from build123d import *

# Parameters (mm, degrees)
BOSS_EXTRUDE1_DEPTH                                  = 3
FILLET1_R                                            = 5
CUT_EXTRUDE1_REACH                                   = 56.362
SKETCH5_W                                            = 36
SKETCH5_H                                            = 28
FILLET2_R                                            = 5
CSK_FOR_M2_5_COUNTERSUNK_FLAT_HEAD_SCREW_D           = 2.7
CSK_FOR_M2_5_COUNTERSUNK_FLAT_HEAD_SCREW_CSINK_D     = 5.5
CSK_FOR_M2_5_COUNTERSUNK_FLAT_HEAD_SCREW_CSINK_ANGLE = 90
CUT_EXTRUDE2_REACH                                   = 56.362
SKETCH3_R                                            = 2.5
MIRROR1_AT_THE_SECOND_PLANE_COPY_1_D                 = 2.7
MIRROR1_AT_THE_SECOND_PLANE_COPY_1_CSINK_D           = 5.5
MIRROR1_AT_THE_SECOND_PLANE_COPY_1_CSINK_ANGLE       = 90
MIRROR1_AT_THE_SECOND_PLANE_COPY_2_REACH             = 56.362
MIRROR1_AT_THE_SECOND_PLANE_COPY_2_SKETC_R           = 2.5
CUT_EXTRUDE3_REACH                                   = 56.362
SKETCH7_R                                            = 1
MIRROR2_AT_THE_SECOND_PLANE_COPY_1_REACH             = 56.362
MIRROR2_AT_THE_SECOND_PLANE_COPY_1_SKETC_R           = 1


with BuildPart() as part:
    # Sketch1 → Boss-Extrude1 (new body)
    with BuildSketch(Plane(origin=(0, 0, 0), x_dir=(1, 0, 0), z_dir=(0, 1, 0))):
        Polygon((8, 26), (-8, 26), (-8, 46.5), (-28, 46.5), (-28, -46.5), (-8, -46.5), (-8, -26), (8, -26), (8, -46.5), (28, -46.5), (28, 46.5), (8, 46.5), align=None)
    extrude(amount=BOSS_EXTRUDE1_DEPTH)

    # Fillet1
    fillet1_edges = [part.edges().sort_by_distance(p)[0] for p in [
        (-8, 1.5, -26),
        (8, 1.5, -26),
        (8, 1.5, -46.5),
        (28, 1.5, -46.5),
        (28, 1.5, 46.5),
        (8, 1.5, 46.5),
        (8, 1.5, 26),
        (-8, 1.5, 26),
        (-8, 1.5, 46.5),
        (-28, 1.5, 46.5),
        (-28, 1.5, -46.5),
        (-8, 1.5, -46.5),
    ]]
    fillet(fillet1_edges, radius=FILLET1_R)

    # Sketch5 → Cut-Extrude1 (cut, up to next)
    with BuildSketch(Plane(origin=(0, 3, 0), x_dir=(1, 0, 0), z_dir=(0, 1, 0)), mode=Mode.PRIVATE) as cut_extrude1_sk1:
        Rectangle(SKETCH5_W, SKETCH5_H)
    cut_extrude1_tool1 = extrude(cut_extrude1_sk1.sketch, amount=-CUT_EXTRUDE1_REACH, mode=Mode.PRIVATE) & part.part
    add(cut_extrude1_tool1.solids().sort_by_distance((0, 3, 0))[0], mode=Mode.SUBTRACT)

    # Fillet2
    fillet2_edges = [part.edges().sort_by_distance(p)[0] for p in [
        (-18, 1.5, 14),
        (-18, 1.5, -14),
        (18, 1.5, -14),
        (18, 1.5, 14),
    ]]
    fillet(fillet2_edges, radius=FILLET2_R)

    # CSK for M2.5 Countersunk Flat Head Screw1 (through all)
    with Locations(Plane(origin=(-18, 3, -37), x_dir=(0, 0, 1), z_dir=(0, 1, 0))):
        with Locations((0, 0), (14, 0)):
            csk_for_m2_5_countersunk_flat_head_screw = CounterSinkHole(CSK_FOR_M2_5_COUNTERSUNK_FLAT_HEAD_SCREW_D / 2, CSK_FOR_M2_5_COUNTERSUNK_FLAT_HEAD_SCREW_CSINK_D / 2, counter_sink_angle=CSK_FOR_M2_5_COUNTERSUNK_FLAT_HEAD_SCREW_CSINK_ANGLE)

    # Sketch3 → Cut-Extrude2 (cut, up to next)
    with BuildSketch(Plane(origin=(0, 3, 0), x_dir=(1, 0, 0), z_dir=(0, 1, 0)), mode=Mode.PRIVATE) as cut_extrude2_sk1:
        with Locations(Location((-18, 30, 0), (0, 0, 270))):
            Circle(SKETCH3_R)
    cut_extrude2_tool1 = extrude(cut_extrude2_sk1.sketch, amount=-CUT_EXTRUDE2_REACH, mode=Mode.PRIVATE) & part.part
    cut_extrude2 = cut_extrude2_tool1.solids().sort_by_distance((-18, 3, -30))[0]
    add(cut_extrude2, mode=Mode.SUBTRACT)

    # Mirror1: CSK for M2.5 Countersunk Flat Head Screw1, Cut-Extrude2 across plane
    add(csk_for_m2_5_countersunk_flat_head_screw.mirror(Plane(origin=(0, 0, 0), x_dir=(0, 0, 1), z_dir=(1, 0, 0))), mode=Mode.SUBTRACT)
    add(cut_extrude2.mirror(Plane(origin=(0, 0, 0), x_dir=(0, 0, 1), z_dir=(1, 0, 0))), mode=Mode.SUBTRACT)

    # Mirror1 at the second plane: CSK for M2.5 Countersunk Flat Head Screw1, Cut-Extrude2 across plane
    add(csk_for_m2_5_countersunk_flat_head_screw.mirror(Plane.XY), mode=Mode.SUBTRACT)
    add(cut_extrude2.mirror(Plane.XY), mode=Mode.SUBTRACT)

    # Mirror1 at the second plane copy 1 (through all)
    with Locations(Plane(origin=(18, 3, 37), x_dir=(0, 0, -1), z_dir=(0, 1, 0))):
        with Locations((0, 0), (14, 0)):
            CounterSinkHole(MIRROR1_AT_THE_SECOND_PLANE_COPY_1_D / 2, MIRROR1_AT_THE_SECOND_PLANE_COPY_1_CSINK_D / 2, counter_sink_angle=MIRROR1_AT_THE_SECOND_PLANE_COPY_1_CSINK_ANGLE)

    # Mirror1 at the second plane copy 2 sketc → Mirror1 at the second plane copy 2 (cut, up to next)
    with BuildSketch(Plane(origin=(0, 3, 0), x_dir=(-1, 0, 0), z_dir=(0, 1, 0)), mode=Mode.PRIVATE) as mirror1_at_the_second_plane_copy_2_sk1:
        with Locations(Location((-18, 30, 0), (0, 0, 270))):
            Circle(MIRROR1_AT_THE_SECOND_PLANE_COPY_2_SKETC_R)
    mirror1_at_the_second_plane_copy_2_tool1 = extrude(mirror1_at_the_second_plane_copy_2_sk1.sketch, amount=-MIRROR1_AT_THE_SECOND_PLANE_COPY_2_REACH, mode=Mode.PRIVATE) & part.part
    add(mirror1_at_the_second_plane_copy_2_tool1.solids().sort_by_distance((18, 3, 30))[0], mode=Mode.SUBTRACT)

    # Sketch7 → Cut-Extrude3 (cut, up to next)
    with BuildSketch(Plane(origin=(0, 3, 0), x_dir=(1, 0, 0), z_dir=(0, 1, 0)), mode=Mode.PRIVATE) as cut_extrude3_sk1:
        with Locations(Location((-23.3, 10, 0), (0, 0, 270))):
            Circle(SKETCH7_R)
    cut_extrude3_tool1 = extrude(cut_extrude3_sk1.sketch, amount=-CUT_EXTRUDE3_REACH, mode=Mode.PRIVATE) & part.part
    cut_extrude3 = cut_extrude3_tool1.solids().sort_by_distance((-23.3, 3, -10))[0]
    add(cut_extrude3, mode=Mode.SUBTRACT)

    # Mirror2: Cut-Extrude3 across plane
    add(cut_extrude3.mirror(Plane(origin=(0, 0, 0), x_dir=(0, 0, 1), z_dir=(1, 0, 0))), mode=Mode.SUBTRACT)

    # Mirror2 at the second plane: Cut-Extrude3 across plane
    add(cut_extrude3.mirror(Plane.XY), mode=Mode.SUBTRACT)

    # Mirror2 at the second plane copy 1 sketc → Mirror2 at the second plane copy 1 (cut, up to next)
    with BuildSketch(Plane(origin=(0, 3, 0), x_dir=(-1, 0, 0), z_dir=(0, 1, 0)), mode=Mode.PRIVATE) as mirror2_at_the_second_plane_copy_1_sk1:
        with Locations(Location((-23.3, 10, 0), (0, 0, 270))):
            Circle(MIRROR2_AT_THE_SECOND_PLANE_COPY_1_SKETC_R)
    mirror2_at_the_second_plane_copy_1_tool1 = extrude(mirror2_at_the_second_plane_copy_1_sk1.sketch, amount=-MIRROR2_AT_THE_SECOND_PLANE_COPY_1_REACH, mode=Mode.PRIVATE) & part.part
    add(mirror2_at_the_second_plane_copy_1_tool1.solids().sort_by_distance((23.3, 3, 10))[0], mode=Mode.SUBTRACT)


solid = part.part
Verification items for the finished model (mm, model axes). A direction names the side the tool comes from. Round coordinates to 2 decimals unless told otherwise and drop trailing zeros. Write each loop counter-clockwise with the first axis right and the second up, starting at its lowest first coordinate (ties: lowest second). Pieces come first, ordered by that corner, then holes.
(1) Section check D-D (y = 1.05). Give the number of separate pieces and of enclosed holes in the cut face, plus the area to 3 significant figures.
Returned:
separate pieces: 1
enclosed holes: 17
area: 3,410 mm2
(2) Access from +Z, -Z, +X, -X, +Y, -Y to the whole of each face (thin tool, end or side, straight path). Record for faces 4 (the cylindrical face through (-26.57, 1.52, 45)), 5 (the flat face through (18, 2, 0)), 6 (the flat face through (0, 1, 26)).
Returned:
face 4: +Z, -X, +Y, -Y
face 5: +Y, -Y
face 6: +Z, +Y, -Y
(3) Material ranges on line 1 (X direction, y = 0.35, z = 37); line 2 (X direction, y = 1.1, z = 23); line 3 (Z direction, x = 7, y = 0.75), recorded low to high.
Returned:
line 1: x = -28 to -19.35, -16.65 to -8, 8 to 16.65, 19.35 to 28
line 2: x = -28 to -19.35, -16.65 to 16.65, 19.35 to 28
line 3: z = -28 to -14, 14 to 28
(4) Section check B-B (x = 0). Enter the section's corners in (y, z).
Returned:
outline: (0, -26) - (3, -26) - (3, -14) - (0, -14) - close; (0, 14) - (3, 14) - (3, 26) - (0, 26) - close
(5) Mould release check, pull along Z, two halves, no side actions. Record for faces 1 (the cylindrical face through (-17.9, 1.5, 32.5)), 2 (the flat face through (8, 1, 36)), 3 (the cylindrical face through (6, 2, 27)): pulls with the +Z half, pulls with the -Z half, needs draft (parallel to the pull), parting line crosses it, or undercut.
Returned:
face 1: undercut
face 2: needs draft
face 3: pulls with the +Z half
(6) Depth check by flat-ended pin: pin 1 Ø3 at (x, z) = (18, -30) entering from -Y; pin 2 Ø1.5 at (x, y) = (-1.5, 1.5) entering from -Z; pin 3 Ø0.9 at (x, y) = (0, 1.5) entering from +Z. Enter the tip coordinate at first touch or a pass-through.
Returned:
pin 1: passes through
pin 2: stops at z = -26
pin 3: stops at z = 26
(7) Section check A-A (z = -37). Enter the section's corners in (x, y), plus the area to 3 significant figures.
Returned:
outline: (-28, 0) - (-19.35, 0) - (-19.35, 1.6) - (-20.75, 3) - (-28, 3) - close; (-16.65, 0) - (-8, 0) - (-8, 3) - (-15.25, 3) - (-16.65, 1.6) - close; (8, 0) - (16.65, 0) - (16.65, 1.6) - (15.25, 3) - (8, 3) - close; (19.35, 0) - (28, 0) - (28, 3) - (20.75, 3) - (19.35, 1.6) - close
area: 99.9 mm2
(8) Section check C-C (z = 2). Enter the section's corners in (x, y), plus the area to 3 significant figures.
Returned:
outline: (-28, 0) - (-18, 0) - (-18, 3) - (-28, 3) - close; (18, 0) - (28, 0) - (28, 3) - (18, 3) - close
area: 60.0 mm2
